Verification items for this drawing (mm, ordinates from the low corner). A direction names the side the tool comes from. Round coordinates to 2 decimals unless told otherwise and drop trailing zeros. Order: outer loops, then holes, each group sorted by start corner. A loop starts at its lowest first (then second) coordinate and runs counter-clockwise, first axis right, second up. Notation, with made-up numbers: (-9.75, 14) -> (43.25, 14) arc R27 cw to (43.25, 47) -> close; hole circle Ø8 at (-34, -25). An arc over 180 degrees is marked (long way). Use a Markdown table: item, result. Add a question column.
Item 1: Sectioned sample at A-A, the plane x = 20.5. Record the cut outline in (y, z).
Item 2: Gauge pin test, flat ends, axial feed: pin 1 Ø10 at (x, z) = (42, 33.5) entering from -Y; pin 2 Ø1 at (x, z) = (11, 35.5) entering from +Y; pin 3 Ø4 at (x, z) = (29, 47) entering from +Y (1 decimal). Record the tip position at first contact, or that the pin passes through.
Item 3: Sectioned sample at C-C, the plane y = 23. Record the cut outline in (x, z) (1 decimal), and give its area (3 significant figures).
Item 4: Material ranges on probe 1 along Z at (x, y) = (32.5, 12); probe 2 along X at (y, z) = (11, 43) (1 decimal); probe 3 along Y at (x, z) = (23.65, 54.5) (1 decimal), recorded low to high. Write a range as [from, to].
Item 5: Mould release check, pull along Y, two halves, no side actions. Record for the marked faces 1, 2 and 3: pulls with the +Y half, pulls with the -Y half, needs draft (parallel to the pull), parting line crosses it, or undercut.
Item 6: Set-up check for the marked faces 4 and 5: record each of +Z, -Z, +X, -X, +Y, -Y from which the full face is reachable in a straight line by a thin tool's end or side.
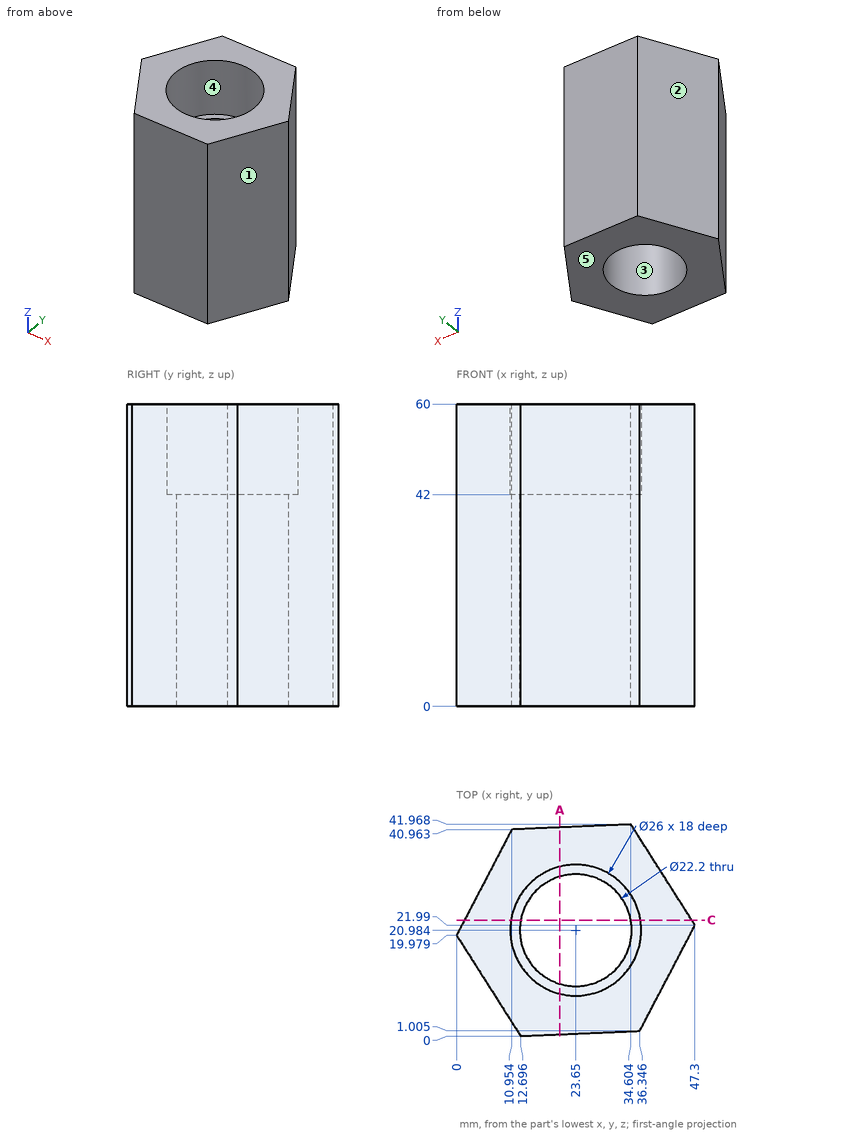
Found:
| question | item | result |
|---|---|---|
| 1 | outline | (0.33, 0) -> (10.34, 0) -> (10.34, 42) -> (8.37, 42) -> (8.37, 60) -> (0.33, 60) -> close; (31.63, 0) -> (41.37, 0) -> (41.37, 60) -> (33.6, 60) -> (33.6, 42) -> (31.63, 42) -> close |
| 2 | pin 1 | stops at y = 2.26 |
| 2 | pin 2 | stops at y = 40.99 |
| 2 | pin 3 | stops at y = 41.8 |
| 3 | outline | (1.6, 0) -> (12.7, 0) -> (12.7, 42) -> (10.8, 42) -> (10.8, 60) -> (1.6, 60) -> close; (34.6, 0) -> (46.7, 0) -> (46.7, 60) -> (36.5, 60) -> (36.5, 42) -> (34.6, 42) -> close |
| 3 | area | 1,330 mm2 |
| 4 | probe 1 | z = [0, 42] |
| 4 | probe 2 | x = [5.7, 15.3], [32, 41.6] |
| 4 | probe 3 | y = [0.5, 8], [34, 41.5] |
| 5 | face 1 | pulls with the -Y half |
| 5 | face 2 | pulls with the +Y half |
| 5 | face 3 | undercut |
| 6 | face 4 | +Z |
| 6 | face 5 | -Z, +X, -X, +Y, -Y |
